Could you check a few things on this model? Use its own coordinates, in mm. Coordinates: 2 decimals unless noted, no trailing zeros. Write each loop counter-clockwise with the first axis right and the second up, starting at its lowest first coordinate (ties: lowest second). Pieces come first, ordered by that corner, then holes. Notation, with made-up numbers: M 64.5,-16.5 L 68.5,-16.5 A28 ccw 68.5,5.5 Z; hole C 57,-15 d11. An arc over 180 degrees is marked long. Answer as CSV lines item,"result". Start each with the question number.
Item 1: I'm going to push flat-ended pins straight in: P1, Ø1.5, axis at x = 23, y = 2.5, coming from the -Z side; P2, Ø3, axis at x = -4, z = 37.5, coming from the -Y side. Where does each tip first touch, or does it pass through?
Item 2: Suppose I cut it at A-A, the plane y = 0.95. Write out the boundary of the cut face in (x, z), and give its area (3 significant figures).
Item 3: Suppose I cut it at B-B, the plane x = 34. Write out the boundary of the cut face in (y, z).
Item 4: If I drill on line 1 along Z through (x, y) = (40, 1.75); line 2 along X through (y, z) = (2.7, 52.5); line 3 along Z through (x, y) = (-42, 2.1), over which ranges is the centre line in solid material (lowest first)? Write a range as [from, to].
Item 5: Suppose I cut it at C-C, the plane z = 38. Write out the boundary of the cut face in (x, y), and give its area (3 significant figures).
```python
from build123d import *

# Parameters (mm, degrees)
EXTRUDE_1_DEPTH = 3
FILLET_1_R      = 15.5


with BuildPart() as part:
    # 草图1 → 凸台-拉伸1 (new body)
    with BuildSketch(Plane(origin=(0, 0, 0), x_dir=(1, 0, 0), z_dir=(0, 1, 0))):
        Polygon((24.852813742, 60), (-24.852813742, 60), (-60, 24.852813742), (-60, -24.852813742), (-24.852813742, -60), (24.852813742, -60), (60, -24.852813742), (60, 24.852813742), align=None)
    extrude(amount=EXTRUDE_1_DEPTH)

    # 圆角1
    fillet_1_edges = [part.edges().sort_by_distance(p)[0] for p in [
        (-60, 1.5, -24.852813742),
        (-24.852813742, 1.5, -60),
        (24.852813742, 1.5, -60),
        (60, 1.5, 24.852813742),
        (-24.852813742, 1.5, 60),
        (-60, 1.5, 24.852813742),
        (24.852813742, 1.5, 60),
        (60, 1.5, -24.852813742),
    ]]
    fillet(fillet_1_edges, radius=FILLET_1_R)


solid = part.part
```
Ans:
1,P1,"stops at z = -59.52"
1,P2,"stops at y = 0"
2,outline,"M -60,-18.43 A15.5 ccw -55.46,-29.39 L -29.39,-55.46 A15.5 ccw -18.43,-60 L 18.43,-60 A15.5 ccw 29.39,-55.46 L 55.46,-29.39 A15.5 ccw 60,-18.43 L 60,18.43 A15.5 ccw 55.46,29.39 L 29.39,55.46 A15.5 ccw 18.43,60 L -18.43,60 A15.5 ccw -29.39,55.46 L -55.46,29.39 A15.5 ccw -60,18.43 Z"
2,area,"11,900 mm^2"
3,outline,"M 0,-50.85 L 3,-50.85 L 3,50.85 L 0,50.85 Z"
4,line 1,"z = [-44.85, 44.85]"
4,line 2,"x = [-32.35, 32.35]"
4,line 3,"z = [-42.85, 42.85]"
5,outline,"M -46.85,0 L 46.85,0 L 46.85,3 L -46.85,3 Z"
5,area,"281 mm^2"
